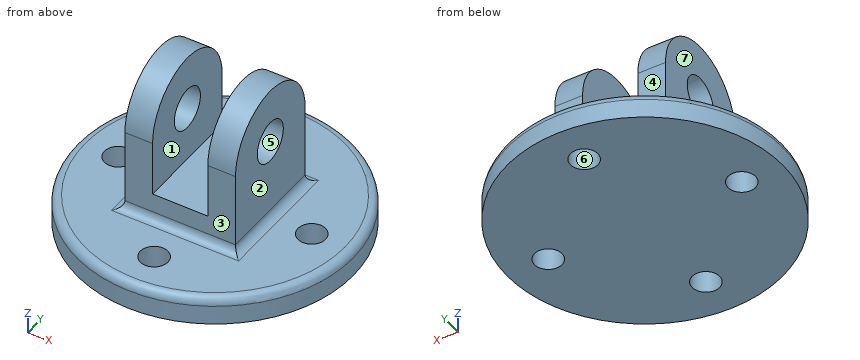
from build123d import *

# Parameters (mm, degrees)
F0_R      = 63.5
F1_DEPTH  = 6.35
F2_R      = 6.35
F3_DEPTH  = 12.701
F5_DEPTH  = 25.4
F7_DEPTH  = 12.7
F8_R      = 9.525
F9_DEPTH  = 12.7
F10_DEPTH = 88.901
F11_R     = 3.81


with BuildPart() as f1:
    # F0 (on Top) → F1 (new body, symmetric)
    with BuildSketch(Plane.XY):
        Circle(F0_R)
    extrude(amount=F1_DEPTH, both=True)

    # F2 (on face) → F3 (cut, through all)
    with BuildSketch(Plane.XY.offset(6.35)):
        with Locations((0, 44.45)):
            Circle(F2_R)
        with Locations((44.45, 0)):
            Circle(F2_R)
        with Locations((0, -44.45)):
            Circle(F2_R)
        with Locations((-44.45, 0)):
            Circle(F2_R)
    extrude(amount=-F3_DEPTH, mode=Mode.SUBTRACT)

    # F4 (on Front) → F5 (join, symmetric)
    with BuildSketch(Plane.XZ):
        Polygon((12.7, 19.05), (-12.7, 19.05), (-12.7, 44.45), (-25.4, 44.45), (-25.4, 6.35), (25.4, 6.35), (25.4, 44.45), (12.7, 44.45), align=None)
    extrude(amount=F5_DEPTH, both=True)

    # F6 (on face) → F7 (join)
    with BuildSketch(Plane.YZ.offset(25.4)):
        with BuildLine():
            Line((-25.4, 44.45), (25.4, 44.45))
            ThreePointArc((25.4, 44.45), (0, 69.85), (-25.4, 44.45))
        make_face()
    extrude(amount=-F7_DEPTH)

    # F8 (on face) → F9 (join)
    with BuildSketch(Plane(origin=(-25.4, 0, 0), x_dir=(0, -1, 0), z_dir=(-1, 0, 0))):
        with Locations((0, 44.45)):
            Circle(F8_R)
        with BuildLine():
            Line((9.525, 44.45), (25.4, 44.45))
            ThreePointArc((25.4, 44.45), (0, 69.85), (-25.4, 44.45))
            Line((-25.4, 44.45), (-9.525, 44.45))
            ThreePointArc((-9.525, 44.45), (0, 53.975), (9.525, 44.45))
        make_face()
    extrude(amount=-F9_DEPTH)

    # F8 (on face) → F10 (cut, through all)
    with BuildSketch(Plane(origin=(-25.4, 0, 0), x_dir=(0, -1, 0), z_dir=(-1, 0, 0))):
        with BuildLine():
            Line((-9.525, 44.45), (9.525, 44.45))
            ThreePointArc((9.525, 44.45), (0, 53.975), (-9.525, 44.45))
        make_face()
        with BuildLine():
            ThreePointArc((-9.525, 44.45), (0, 34.925), (9.525, 44.45))
            Line((9.525, 44.45), (-9.525, 44.45))
        make_face()
    extrude(amount=-F10_DEPTH, mode=Mode.SUBTRACT)

    # F11
    f11_edges = [f1.edges().sort_by_distance(p)[0] for p in [
        (0, -25.4, 6.35),
        (-25.4, 0, 6.35),
        (0, 25.4, 6.35),
        (25.4, 0, 6.35),
        (-63.5, 0, 6.35),
    ]]
    fillet(f11_edges, radius=F11_R)


solid = f1.part
Geometry: final body of the model. Coordinates: model frame, mm. Face numbers are marked on the shaded views. A direction names the side the tool comes from. Coordinates: 2 decimals unless noted, no trailing zeros. Order: outer loops, then holes, each group sorted by start corner. A loop starts at its lowest first (then second) coordinate and runs counter-clockwise, first axis right, second up. Notation, with made-up numbers: M 36,64 L 67,64 A26 ccw 67,102 Z; hole C -18.5,-20.5 d7. An arc over 180 degrees is marked long. One line per question, with ' | ' between items. Start each with the question number.
Item 1: Cut plane D-D, the plane z = 8. Return the cut outline in (x, y).
Item 2: Cut plane C-C, the plane z = 37.5. Return the cut outline in (x, y), then the cut area to 3 significant figures.
Item 3: Draft query along X for the marked faces 5, 6 and 7. Return one class per face: released by +X, released by -X, zero draft, split by the parting line, or undercut.
Item 4: Cut plane A-A, the plane y = 0. Count the separate pieces of the cut face and the enclosed holes in it, then the cut area to 3 significant figures.
Item 5: Set-up query: the marked faces 1, 2, 3 and 4. Return all of +Z, -Z, +X, -X, +Y, -Y with unobstructed straight access to the full face (end or side cutting, diameter ignored); none if empty.
Item 6: Pin query (flat end, axial travel): pin 1 Ø4 at (y, z) = (16, 61) entering from -X; pin 2 Ø16.5 at (x, y) = (44.45, 0) entering from +Z; pin 3 Ø15 at (y, z) = (-3, 50.5) entering from +X; pin 4 Ø17 at (y, z) = (0, 44.45) entering from +X. Return the tip coordinate at first contact, or that it passes through.
Item 7: Ray query, probe 1 along Y at (x, z) = (0, 1); probe 2 along X at (y, z) = (-3, 64); probe 3 along Y at (x, z) = (-19, 44). Return the intervals inside material, ascending. Write a range as [from, to].
Item 8: Cut plane B-B, the plane x = 0. Return the cut outline in (y, z), then the cut area to 3 significant figures.
A:
1) outline: M -26.07,-26.07 L 26.07,-26.07 L 26.07,26.07 L -26.07,26.07 Z
2) outline: M -25.4,-25.4 L -12.7,-25.4 L -12.7,-6.51 L -25.4,-6.51 Z; M -25.4,6.51 L -12.7,6.51 L -12.7,25.4 L -25.4,25.4 Z; M 12.7,-25.4 L 25.4,-25.4 L 25.4,-6.51 L 12.7,-6.51 Z; M 12.7,6.51 L 25.4,6.51 L 25.4,25.4 L 12.7,25.4 Z | area: 959 mm2
3) face 5: zero draft | face 6: undercut | face 7: released by -X
4) separate pieces: 5 | enclosed holes: 0 | area: 2,740 mm2
5) face 1: +Z, +Y, -Y | face 2: +Z, +X, +Y, -Y | face 3: +Z, +X, -X, -Y | face 4: +Z, +X, -X, +Y
6) pin 1: stops at x = -25.4 | pin 2: stops at z = 6.35 | pin 3: stops at x = 25.4 | pin 4: passes through
7) probe 1: y = [-63.5, -50.8], [-38.1, 38.1], [50.8, 63.5] | probe 2: x = [-25.4, -12.7], [12.7, 25.4] | probe 3: y = [-25.4, -9.51], [9.51, 25.4]
8) outline: M -63.5,-6.35 L -50.8,-6.35 L -50.8,6.35 L -59.69,6.35 A3.81 ccw -63.5,2.54 Z; M -38.1,-6.35 L 38.1,-6.35 L 38.1,6.35 L 29.21,6.35 A3.81 cw 25.4,10.16 L 25.4,19.05 L -25.4,19.05 L -25.4,10.16 A3.81 cw -29.21,6.35 L -38.1,6.35 Z; M 50.8,-6.35 L 63.5,-6.35 L 63.5,2.54 A3.81 ccw 59.69,6.35 L 50.8,6.35 Z | area: 1,940 mm2
